Verification items for this drawing (mm, ordinates from the low corner). Give positions to 0.01 mm unless a question says otherwise; leave off trailing zeros. One line per question, with ' | ' between items.
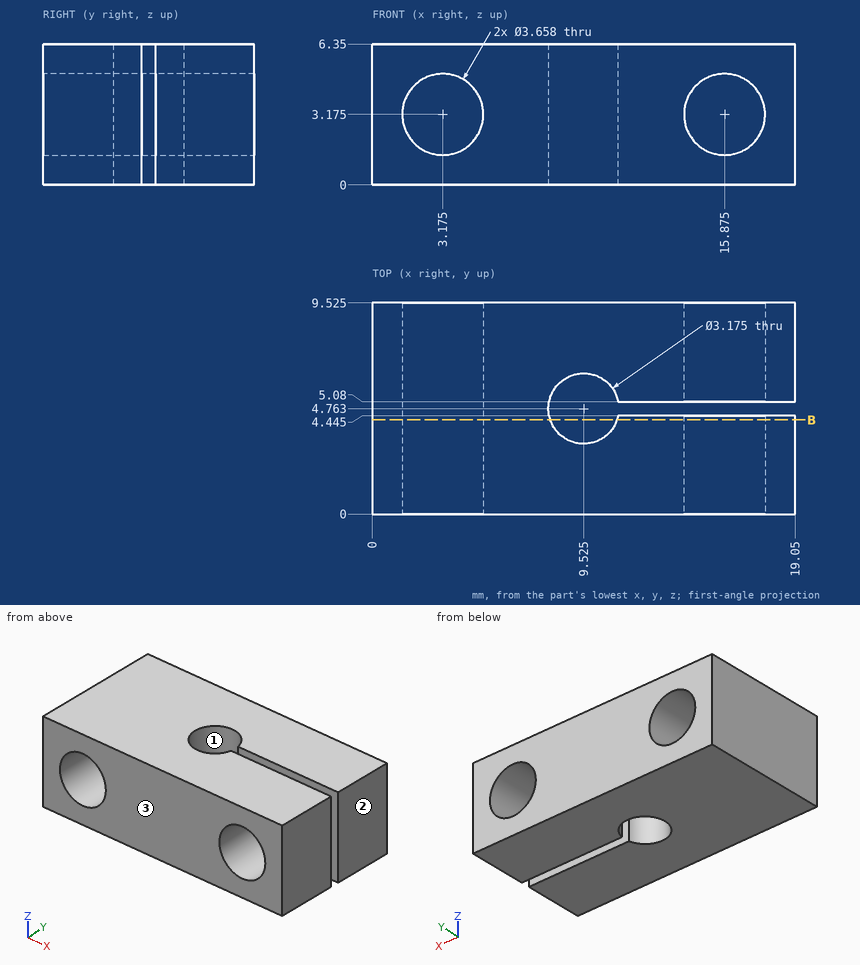
Q1. Mould release check, pull along Y, two halves, no side actions. Record for the marked faces 1, 2 and 3: pulls with the +Y half, pulls with the -Y half, needs draft (parallel to the pull), parting line crosses it, or undercut.
Result sheet:
face 1: undercut | face 2: needs draft | face 3: pulls with the -Y half
Q2. Depth check by flat-ended pin: pin 1 Ø2 at (x, z) = (15.875, 3.175) entering from +Y. Enter the tip coordinate at first touch or a pass-through.
Result sheet:
pin 1: passes through
Q3. Thickness scan on line 1 (X direction, y = 1, z = 3.25); line 2 (Y direction, x = 17, z = 5) (1 decimal); line 3 (Z direction, x = 3.25, y = 2.25). Record the ranges inside material, lowest first.
Result sheet:
line 1: x = 0 to 1.35, 5 to 14.05, 17.7 to 19.05 | line 2: y = 0 to 4.4, 5.1 to 9.5 | line 3: z = 0 to 1.35, 5 to 6.35
Q4. Section check B-B (y = 4.25). Count the separate pieces of the cut face and the enclosed holes in it.
Result sheet:
separate pieces: 2 | enclosed holes: 2
